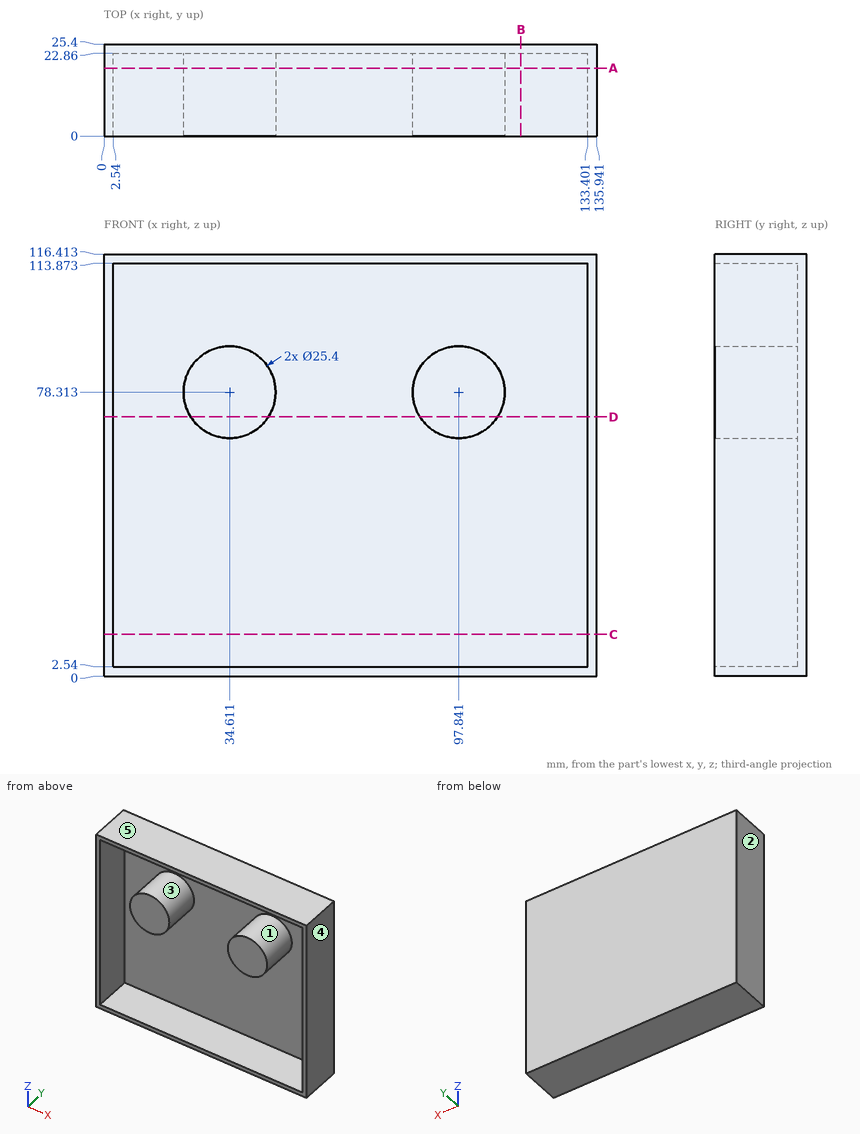
Could you check a few things on this drawing? It's one solid part, dimensions in mm from its lowest x, y, z. A direction names the side the tool comes from. Give positions to 0.01 mm unless a question says otherwise; leave off trailing zeros. Order: outer loops, then holes, each group sorted by start corner. A loop starts at its lowest first (then second) coordinate and runs counter-clockwise, first axis right, second up. Notation, with made-up numbers: (21.25, 79.5) - (55.25, 79.5) arc R27 ccw to (55.25, 104.5) - close; hole circle Ø10 at (45.5, 82). An arc over 180 degrees is marked (long way). One line per question, with ' | ' between items. Start each with the question number.
Item 1: I need wall thicknesses on probe 1 along Z at (x, y) = (33.5, 3.25) (1 decimal); probe 2 along Z at (x, y) = (115.5, 11.75); probe 3 along X at (y, z) = (19, 86). Which ranges of each line are inside material? Lowest first, please. Write a range as [from, to].
Item 2: I want a section at B-B on x = 115. Write out the boundary of the cut face in (y, z).
Item 3: For the marked faces 1 and 2, which set-ups out of +Z, -Z, +X, -X, +Y, -Y let a thin tool reach every point of the face, with its end or its side?
Item 4: I want a section at D-D on z = 71.5. Write out the boundary of the cut face in (x, y), then the cut area to 3 significant figures.
Item 5: I want a section at A-A on y = 18.75. Write out the boundary of the cut face in (x, z), then the cut area to 3 significant figures.
Item 6: I'm going to push a flat-ended pin straight in: pin 1 Ø5 at (x, z) = (69.5, 31) entering from -Y. Where does the tip first touch, or does it pass through?
Item 7: Thinking about a two-plate mould opening in Z: for the marked faces 3, 4 and 5, which applies, pulls with the +Z half, pulls with the -Z half, needs draft (parallel to the pull), parting line crosses it, or undercut?
Item 8: I want a section at C-C on z = 11.5. Write out the boundary of the cut face in (x, y).
Verdict:
1) probe 1: [0, 2.5], [65.7, 91], [113.9, 116.4] | probe 2: [0, 2.54], [113.87, 116.41] | probe 3: [0, 2.54], [24.5, 44.72], [87.73, 107.95], [133.4, 135.94]
2) outline: (0, 0) - (25.4, 0) - (25.4, 116.41) - (0, 116.41) - (0, 113.87) - (22.86, 113.87) - (22.86, 2.54) - (0, 2.54) - close
3) face 1: -Y | face 2: +Z, -Z, -X, +Y, -Y
4) outline: (0, 0) - (2.54, 0) - (2.54, 22.86) - (23.89, 22.86) - (23.89, 0) - (45.33, 0) - (45.33, 22.86) - (87.12, 22.86) - (87.12, 0) - (108.56, 0) - (108.56, 22.86) - (133.4, 22.86) - (133.4, 0) - (135.94, 0) - (135.94, 25.4) - (0, 25.4) - close | area: 1,440 mm^2
5) outline: (0, 0) - (135.94, 0) - (135.94, 116.41) - (0, 116.41) - close; circle Ø25.4 at (34.61, 78.31); circle Ø25.4 at (97.84, 78.31); hole (2.54, 2.54) - (133.4, 2.54) - (133.4, 113.87) - (2.54, 113.87) - close | area: 2,270 mm^2
6) pin 1: y = 22.86
7) face 3: undercut | face 4: needs draft | face 5: pulls with the +Z half
8) outline: (0, 0) - (2.54, 0) - (2.54, 22.86) - (133.4, 22.86) - (133.4, 0) - (135.94, 0) - (135.94, 25.4) - (0, 25.4) - close
